Here's how the part is built. I have some questions about the finished solid (model axes, mm). Round coordinates to 2 decimals unless told otherwise and drop trailing zeros. Loops run counter-clockwise (first coordinate to the right, second up) from the corner with the lowest first, then second, coordinate; pieces in that order, holes last. Notation, with made-up numbers: M 41.5,29.25 L 61.5,29.25 A17 ccw 61.5,38.25 Z; hole C 9.5,55.25 d8. An arc over 180 degrees is marked long. Use a Markdown table: item, result.
from build123d import *

# Parameters (mm, degrees)
F1_DEPTH = 5
F2_DEPTH = 1000


with BuildPart() as f1:
    # F0 (on Top) → F1 (new body)
    with BuildSketch(Plane.XY):
        with BuildLine():
            Line((-5, 100), (-5, 2.8867513459))
            Line((-5, 2.8867513459), (-2.5, 4.3301270189))
            ThreePointArc((-2.5, 4.3301270189), (0, 5), (2.5, 4.3301270189))
            Line((2.5, 4.3301270189), (5, 2.8867513459))
            Line((5, 2.8867513459), (5, 100))
            Line((5, 100), (-5, 100))
        make_face()
        with BuildLine():
            Line((-2.5, 4.3301270189), (-5, 2.8867513459))
            Line((-5, 2.8867513459), (-5, 0))
            ThreePointArc((-5, 0), (-4.3301270189, 2.5), (-2.5, 4.3301270189))
        make_face()
        with BuildLine():
            Line((-89.1025403784, -45.6698729811), (-86.6025403784, -50))
            Line((-86.6025403784, -50), (-84.1025403784, -54.3301270189))
            Line((-84.1025403784, -54.3301270189), (0, -5.7735026919))
            Line((0, -5.7735026919), (-2.5, -4.3301270189))
            ThreePointArc((-2.5, -4.3301270189), (-4.3301270189, -2.5), (-5, 0))
            Line((-5, 0), (-5, 2.8867513459))
            Line((-5, 2.8867513459), (-89.1025403784, -45.6698729811))
        make_face()
        with BuildLine():
            Line((-2.5, -4.3301270189), (0, -5.7735026919))
            Line((0, -5.7735026919), (2.5, -4.3301270189))
            ThreePointArc((2.5, -4.3301270189), (0, -5), (-2.5, -4.3301270189))
        make_face()
        with BuildLine():
            Line((2.5, -4.3301270189), (0, -5.7735026919))
            Line((0, -5.7735026919), (84.1025403784, -54.3301270189))
            Line((84.1025403784, -54.3301270189), (86.6025403784, -50))
            Line((86.6025403784, -50), (89.1025403784, -45.6698729811))
            Line((89.1025403784, -45.6698729811), (5, 2.8867513459))
            Line((5, 2.8867513459), (5, 0))
            ThreePointArc((5, 0), (4.3301270189, -2.5), (2.5, -4.3301270189))
        make_face()
        with BuildLine():
            Line((5, 2.8867513459), (2.5, 4.3301270189))
            ThreePointArc((2.5, 4.3301270189), (4.3301270189, 2.5), (5, 0))
            Line((5, 0), (5, 2.8867513459))
        make_face()
    extrude(amount=F1_DEPTH)

    # F0 (on Top) → F2 (join)
    with BuildSketch(Plane.XY):
        with BuildLine():
            Line((2.5, 4.3301270189), (0, 0))
            Line((0, 0), (5, 0))
            ThreePointArc((5, 0), (4.3301270189, 2.5), (2.5, 4.3301270189))
        make_face()
        with BuildLine():
            Line((0, 0), (2.5, -4.3301270189))
            ThreePointArc((2.5, -4.3301270189), (4.3301270189, -2.5), (5, 0))
            Line((5, 0), (0, 0))
        make_face()
        with BuildLine():
            ThreePointArc((-2.5, -4.3301270189), (0, -5), (2.5, -4.3301270189))
            Line((2.5, -4.3301270189), (0, 0))
            Line((0, 0), (-2.5, -4.3301270189))
        make_face()
        with BuildLine():
            Line((0, 0), (-5, 0))
            ThreePointArc((-5, 0), (-4.3301270189, -2.5), (-2.5, -4.3301270189))
            Line((-2.5, -4.3301270189), (0, 0))
        make_face()
        with BuildLine():
            Line((0, 0), (-2.5, 4.3301270189))
            ThreePointArc((-2.5, 4.3301270189), (-4.3301270189, 2.5), (-5, 0))
            Line((-5, 0), (0, 0))
        make_face()
        with BuildLine():
            ThreePointArc((2.5, 4.3301270189), (0, 5), (-2.5, 4.3301270189))
            Line((-2.5, 4.3301270189), (0, 0))
            Line((0, 0), (2.5, 4.3301270189))
        make_face()
    extrude(amount=F2_DEPTH)


solid = f1.part
1. Imagine slicing it at C-C, the plane x = -69. Write out the boundary of the cut face in (y, z).
Answer sheet:
| item | result |
|---|---|
| outline | M -45.61,0 L -34.06,0 L -34.06,5 L -45.61,5 Z |
2. Imagine slicing it at A-A, the plane y = -20. Write out the boundary of the cut face in (x, z), then the cut area to 3 significant figures.
Answer sheet:
| item | result |
|---|---|
| outline | M -44.64,0 L -24.64,0 L -24.64,5 L -44.64,5 Z; M 24.64,0 L 44.64,0 L 44.64,5 L 24.64,5 Z |
| area | 200 mm2 |
3. We'd pull the mould along X, two halves only. Please class faces 1 (the face through (-46.46, -21.05, 2.46)), 2 (the face through (0, -5, 0)), 3 (the face through (41.46, -29.71, 2.46)), 4 (the face through (47.64, -21.73, 2.46)): +X half, -X half, draft (parallel to the pull), parting line (faces both ways), or undercut.
Answer sheet:
| item | result |
|---|---|
| face 1 | -X half |
| face 2 | draft |
| face 3 | undercut |
| face 4 | +X half |
4. I need wall thicknesses on probe 1 along Z at (x, y) = (-80, -46); probe 2 along Y at (x, z) = (0, 659); probe 3 along Y at (x, z) = (-3, 427). Which ranges of each line are inside material? Lowest first, please. Write a range as from..to.
Answer sheet:
| item | result |
|---|---|
| probe 1 | 0..5 |
| probe 2 | -5..5 |
| probe 3 | -4..4 |
5. Imagine slicing it at D-D, the plane y = 84.5. Write out the boundary of the cut face in (x, z).
Answer sheet:
| item | result |
|---|---|
| outline | M -5,0 L 5,0 L 5,5 L -5,5 Z |
6. Imagine slicing it at B-B, the plane z = 610. Write out the boundary of the cut face in (x, y).
Answer sheet:
| item | result |
|---|---|
| outline | C 0,0 d10 |
7. For pin 1 Ø4 at (y, z) = (29, 3) entering from +X; pin 2 Ø4 at (y, z) = (65, 3) entering from -X; pin 3 Ø6 at (y, z) = (9, 884) entering from +X, each with a flat end and sliding along its axis, tell me the tip position at first contact or that it passes through.
Answer sheet:
| item | result |
|---|---|
| pin 1 | x = 5 |
| pin 2 | x = -5 |
| pin 3 | through |
